Input: dimensioned drawing with shaded views. Units: mm. Origin: part minimum x, y, z. A direction names the side the tool comes from. Give positions to 0.01 mm unless a question says otherwise; leave off trailing zeros. Write each loop counter-clockwise with the first axis right and the second up, starting at its lowest first coordinate (ties: lowest second). Pieces come first, ordered by that corner, then holes. Notation, with made-up numbers: M 59.5,10 L 93.5,10 A14 ccw 93.5,27 Z; hole C 89,-38.5 d5. An arc over 180 degrees is marked long. Answer as a JSON object with one key per item and string values.
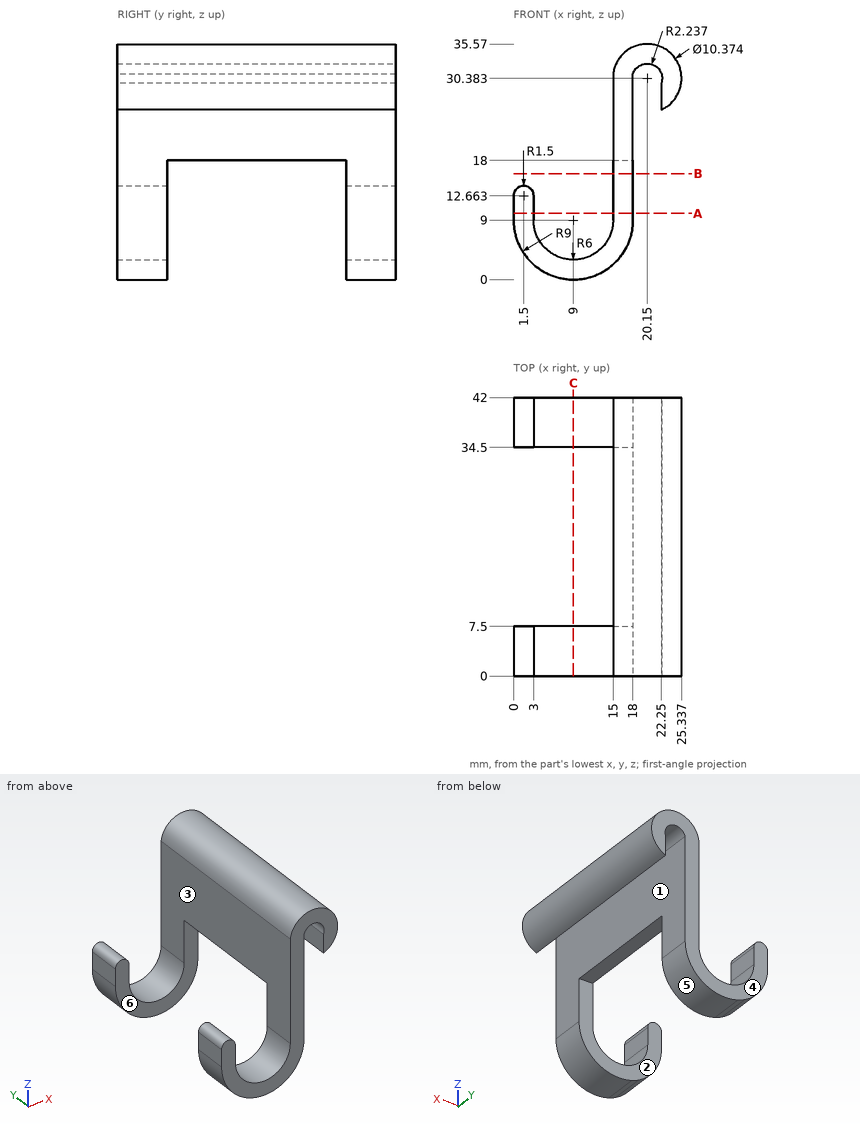
1) Cut plane C-C on x = 9. Return loops of the section in (y, z).
Geometry check:
{"outline": "M 0,0 L 7.5,0 L 7.5,3 L 0,3 Z; M 34.5,0 L 42,0 L 42,3 L 34.5,3 Z"}
2) Contact query for flat-ended pins moving along their axis: P1, Ø11, axis at y = 11.5, z = 25, coming from the +X side; P2, Ø2, axis at y = 29.5, z = 29.5, coming from the -X side; P3, Ø3, axis at y = 40, z = 11, coming from the +X side; P4, Ø6, axis at x = 13.5, y = 16, coming from the +Z side. Output: stop coordinate, or through.
Geometry check:
{"P1": "stops at x = 25.34", "P2": "stops at x = 15", "P3": "stops at x = 18", "P4": "stops at z = 34.07"}
3) Cut plane B-B on z = 16. Return loops of the section in (x, y).
Geometry check:
{"outline": "M 15,0 L 18,0 L 18,7.5 L 15,7.5 Z; M 15,34.5 L 18,34.5 L 18,42 L 15,42 Z"}
4) Cut plane A-A on z = 10. Return loops of the section in (x, y).
Geometry check:
{"outline": "M 0,0 L 3,0 L 3,7.5 L 0,7.5 Z; M 0,34.5 L 3,34.5 L 3,42 L 0,42 Z; M 15,0 L 18,0 L 18,7.5 L 15,7.5 Z; M 15,34.5 L 18,34.5 L 18,42 L 15,42 Z"}
5) Pull-direction query (Y, two-part tool) for the marked faces 4, 5 and 6; classes: pulls with the +Y half, pulls with the -Y half, needs draft (parallel to the pull), parting line crosses it, or undercut.
Geometry check:
{"face 4": "pulls with the +Y half", "face 5": "needs draft", "face 6": "undercut"}
6) Line query: line 1 (Y direction, x = 16.5, z = 14.5); line 2 (X direction, y = 36.5, z = 30); line 3 (X direction, y = 21, z = 32) (1 decimal). Output: solid intervals per line, ascending. Write a range as from..to.
Geometry check:
{"line 1": "y = 0..7.5, 34.5..42", "line 2": "x = 15..18, 22.35..25.32", "line 3": "x = 15.2..18.6, 21.7..25.1"}
7) Set-up query: the marked faces 1, 2 and 3. Return all of +Z, -Z, +X, -X, +Y, -Y with unobstructed straight access to the full face (end or side cutting, diameter ignored); none if empty.
Geometry check:
{"face 1": "-Z, +Y, -Y", "face 2": "-Z, +X, -X", "face 3": "+Z, +Y, -Y"}
